Design review of the part built by this model. Coordinates are the model's own, in mm. Face numbers are marked on the shaded views. A direction names the side the tool comes from. Coordinates: 2 decimals unless noted, no trailing zeros. Order: outer loops, then holes, each group sorted by start corner. A loop starts at its lowest first (then second) coordinate and runs counter-clockwise, first axis right, second up. Notation, with made-up numbers: (64, 53) -> (94, 53) arc R20 cw to (94, 67) -> close; hole circle Ø10 at (32, 26.5). An arc over 180 degrees is marked (long way). Use a Markdown table: item, result. Add a question column.
Q1. Add section D-D (z = -34.5). State the section outline as (x, y) points, then the cut area to 3 significant figures.
Q2. Wall thickness on probe 1 along Z at (x, y) = (1.5, 3.5); probe 2 along Z at (x, y) = (4.25, 2.25); probe 3 along Z at (x, y) = (2, -2.5): over which ranges is each line inside the solid? List them lowest first.
Q3. Insertion check: pin 1 (2 mm diameter, centred on y = 4, z = -15, fed in from +X); pin 2 (1 mm diameter, centred on y = 3, z = -33, fed in from -X); pin 3 (1.5 mm diameter, centred on x = 0.5, z = -25.5, fed in from -Y). Each pin has a flat end and moves straight along its axis. Give the tip position at first contact, or say it passes through.
Q4. Add section C-C (z = -50). State the section outline as (x, y) points, then the cut area to 3 significant figures.
Q5. Add section A-A (x = 0). State the section outline as (y, z) points, then the cut area to 3 significant figures.
Q6. Machinability: for the marked faces 4 and 5, which of the approach directions +Z, -Z, +X, -X, +Y, -Y give a long, thin tool a straight path to every point of the face, cutting with its end or side? Answer none if there is none.
Q7. The part is to be moulded in two halves that separate along Z. For the marked faces 1, 2 and 3, say which applies: pulls with the +Z half, pulls with the -Z half, needs draft (parallel to the pull), parting line crosses it, or undercut.
Autodesk Inventor part; units mm, degrees
ref_plane "YZ Plane" through (0, 0, 0) normal (1, 0, 0) x (0, 1, 0)
ref_plane "XZ Plane" through (0, 0, 0) normal (0, 1, 0) x (-1, 0, 0)
ref_plane "XY Plane" through (0, 0, 0) normal (0, 0, 1) x (1, 0, 0)
sketch "Skizze1" plane through (0, 0, 0) normal (0, 1, 0) x (-1, 0, 0)
  line L0 (0, 0) -> (0, -55)
  line L1 (0, 0) -> (4, 0)
  line L2 (4, 0) -> (4, -8)
  arc A0 (4, -8) -> (4, -10) centre (4, -9) ccw
  line L3 (4, -10) -> (7.5, -10)
  line L4 (7.5, -10) -> (7.5, -15)
  line L5 (7.5, -15) -> (4.7029, -15)
  line L6 (4.7029, -15) -> (7.5, -55)
  line L7 (7.5, -55) -> (0, -55)
  point P0 (2, 0)
  dimension "d0" = 4
  dimension "d1" = 5
  dimension "d2" = 8
  dimension "d3" = 15
  dimension "d4" = 8
  dimension "d5" = 10
  dimension "d6" = 55
  dimension "d7" = 15
revolve "Umdrehung1" add sketch "Skizze1" angle 360 about axis through (0, 0, 0) along (0, 0, -1)
fillet "Rundung1" radius 2 1 edges at (4.7029, 0, -15)
fillet "Rundung2" radius 1 1 edges at (7.5, 0, -55)
properties part number "Griff" material "Stahl, galvanisiert"
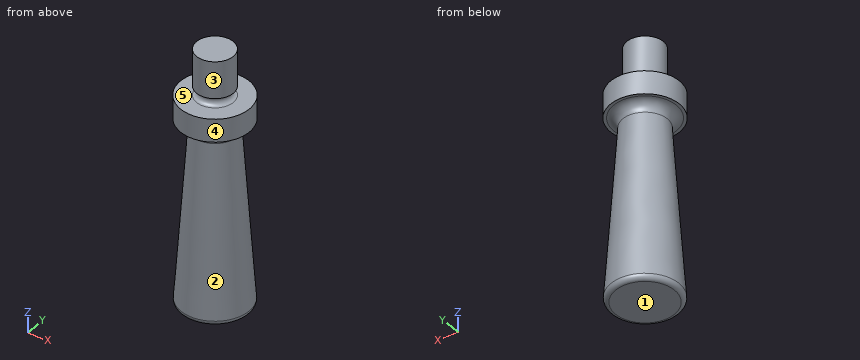
Established:
| question | item | result |
|---|---|---|
| 1 | outline | circle Ø12.13 at (0, 0) |
| 1 | area | 116 mm^2 |
| 2 | probe 1 | -55 to -9.98, -8.02 to 0 |
| 2 | probe 2 | -55 to -10 |
| 2 | probe 3 | -55 to -9.6, -8.4 to 0 |
| 3 | pin 1 | x = 6.87 |
| 3 | pin 2 | x = -5.42 |
| 3 | pin 3 | y = -5.48 |
| 4 | outline | circle Ø14.3 at (0, 0) |
| 4 | area | 161 mm^2 |
| 5 | outline | (-7.5, -15) -> (-6.85, -15) arc R2 cw to (-4.85, -17.14) -> (-7.43, -53.93) arc R1 ccw to (-6.43, -55) -> (6.43, -55) arc R1 ccw to (7.43, -53.93) -> (4.85, -17.14) arc R2 cw to (6.85, -15) -> (7.5, -15) -> (7.5, -10) -> (4, -10) arc R1 cw to (4, -8) -> (4, 0) -> (-4, 0) -> (-4, -8) arc R1 cw to (-4, -10) -> (-7.5, -10) -> close |
| 5 | area | 641 mm^2 |
| 6 | face 4 | +Z, -Z |
| 6 | face 5 | +Z |
| 7 | face 1 | pulls with the -Z half |
| 7 | face 2 | undercut |
| 7 | face 3 | needs draft |
